Can you work these out from the model? Positions are in its coordinate system, mm. A direction names the side the tool comes from. Give positions to 0.01 mm unless a question says otherwise; leave off trailing zeros. Loops run counter-clockwise (first coordinate to the right, second up) from the corner with the lowest first, then second, coordinate; pieces in that order, holes last. Notation, with made-up numbers: (48.25, 86.25) -> (91.25, 86.25) arc R20 cw to (91.25, 118.25) -> close; hole circle Ø9 at (30.25, 83.25). An arc over 180 degrees is marked (long way). One line per question, with ' | ' between items.
from build123d import *

# Parameters (mm, degrees)
SKETCH1_W                                 = 95
SKETCH1_H                                 = 134
BOSS_EXTRUDE1_DEPTH                       = 2
CSK_FOR_4_FLAT_HEAD_MACHINE_SCREW_2_COUNT = 2
CSK_FOR_4_FLAT_HEAD_MACHINE_SCREW_2_PITCH = 46.7
CSK_FOR_4_FLAT_HEAD_MACHINE_SCREW_3_COUNT = 2
CSK_FOR_4_FLAT_HEAD_MACHINE_SCREW_3_PITCH = 55.505765466
CSK_FOR_4_FLAT_HEAD_MACHINE_SCREW_4_COUNT = 2
CSK_FOR_4_FLAT_HEAD_MACHINE_SCREW_4_PITCH = 30
CSK_FOR_4_FLAT_HEAD_MACHINE_SCREW_5_COUNT = 2
CSK_FOR_4_FLAT_HEAD_MACHINE_SCREW_5_PITCH = 116.985137945
CSK_FOR_4_FLAT_HEAD_MACHINE_SCREW_6_COUNT = 2
CSK_FOR_4_FLAT_HEAD_MACHINE_SCREW_6_PITCH = 131.458824352
SKETCH13_R                                = 24.6
CUT_EXTRUDE2_DEPTH                        = 165.271117364
SKETCH14_R                                = 3
BOSS_EXTRUDE4_DEPTH                       = 19.3
SKETCH15_R                                = 1.15
CUT_EXTRUDE3_DEPTH                        = 15
SKETCH16_W                                = 4
SKETCH16_H                                = 14
CUT_EXTRUDE4_DEPTH                        = 166.388905311


with BuildPart() as part:
    # Sketch1 → Boss-Extrude1 (new body)
    with BuildSketch(Plane.XY):
        with Locations((47.5, 67)):
            Rectangle(SKETCH1_W, SKETCH1_H)
    extrude(amount=BOSS_EXTRUDE1_DEPTH)

    # Sketch8 → CSK for #4 Flat Head Machine Screw (100)2 (revolve, cut)
    with BuildSketch(Plane(origin=(70.85, 130, 0), x_dir=(0, 1, 0), z_dir=(1, 0, 0))):
        Polygon((0, 0), (0, 2), (1.63195, 2), (1.63195, 1.028358553), (2.8575, 0), align=None)
    csk_for_4_flat_head_machine_screw_100 = revolve(axis=Axis((70.85, 130, -6.35), (0, 0, 1)), mode=Mode.SUBTRACT)

    # CSK for _4 Flat Head Machine Screw _ 2: CSK for #4 Flat Head Machine Screw (100)2 ×2
    with Locations(*[(-i * CSK_FOR_4_FLAT_HEAD_MACHINE_SCREW_2_PITCH, 0, 0) for i in range(1, CSK_FOR_4_FLAT_HEAD_MACHINE_SCREW_2_COUNT)]):
        add(csk_for_4_flat_head_machine_screw_100, mode=Mode.SUBTRACT)

    # CSK for _4 Flat Head Machine Screw _ 3: CSK for #4 Flat Head Machine Screw (100)2 ×2
    with Locations(*[Vector(-0.8413540396691381, -0.540484393791738, 0) * (i * CSK_FOR_4_FLAT_HEAD_MACHINE_SCREW_3_PITCH) for i in range(1, CSK_FOR_4_FLAT_HEAD_MACHINE_SCREW_3_COUNT)]):
        add(csk_for_4_flat_head_machine_screw_100, mode=Mode.SUBTRACT)

    # CSK for _4 Flat Head Machine Screw _ 4: CSK for #4 Flat Head Machine Screw (100)2 ×2
    with Locations(*[(0, -i * CSK_FOR_4_FLAT_HEAD_MACHINE_SCREW_4_PITCH, 0) for i in range(1, CSK_FOR_4_FLAT_HEAD_MACHINE_SCREW_4_COUNT)]):
        add(csk_for_4_flat_head_machine_screw_100, mode=Mode.SUBTRACT)

    # CSK for _4 Flat Head Machine Screw _ 5: CSK for #4 Flat Head Machine Screw (100)2 ×2
    with Locations(*[Vector(0.12950362982970207, -0.991578947870986, 0) * (i * CSK_FOR_4_FLAT_HEAD_MACHINE_SCREW_5_PITCH) for i in range(1, CSK_FOR_4_FLAT_HEAD_MACHINE_SCREW_5_COUNT)]):
        add(csk_for_4_flat_head_machine_screw_100, mode=Mode.SUBTRACT)

    # CSK for _4 Flat Head Machine Screw _ 6: CSK for #4 Flat Head Machine Screw (100)2 ×2
    with Locations(*[Vector(-0.47048952632046626, -0.8824055788710445, 0) * (i * CSK_FOR_4_FLAT_HEAD_MACHINE_SCREW_6_PITCH) for i in range(1, CSK_FOR_4_FLAT_HEAD_MACHINE_SCREW_6_COUNT)]):
        add(csk_for_4_flat_head_machine_screw_100, mode=Mode.SUBTRACT)

    # Sketch13 → Cut-Extrude2 (cut, through all)
    with BuildSketch(Plane(origin=(0, 0, 0), x_dir=(-1, 0, 0), z_dir=(0, 0, -1))):
        with Locations((-47.5, 45.5)):
            Circle(SKETCH13_R)
    extrude(amount=-CUT_EXTRUDE2_DEPTH, mode=Mode.SUBTRACT)

    # Sketch14 → Boss-Extrude4 (add)
    with BuildSketch(Plane(origin=(0, 0, 0), x_dir=(-1, 0, 0), z_dir=(0, 0, -1))):
        with Locations((-72, 70.1)):
            Circle(SKETCH14_R)
        with Locations((-23, 70.1)):
            Circle(SKETCH14_R)
        with Locations((-72, 20.9)):
            Circle(SKETCH14_R)
        with Locations((-23, 20.9)):
            Circle(SKETCH14_R)
    extrude(amount=BOSS_EXTRUDE4_DEPTH)

    # Sketch15 → Cut-Extrude3 (cut)
    with BuildSketch(Plane(origin=(0, 0, -19.3), x_dir=(-1, 0, 0), z_dir=(0, 0, -1))):
        with Locations((-72, 70.1)):
            Circle(SKETCH15_R)
        with Locations((-23, 70.1)):
            Circle(SKETCH15_R)
        with Locations((-23, 20.9)):
            Circle(SKETCH15_R)
        with Locations((-72, 20.9)):
            Circle(SKETCH15_R)
    extrude(amount=-CUT_EXTRUDE3_DEPTH, mode=Mode.SUBTRACT)

    # Sketch16 → Cut-Extrude4 (cut, through all)
    with BuildSketch(Plane(origin=(0, 0, 0), x_dir=(-1, 0, 0), z_dir=(0, 0, -1))):
        with Locations((-19, 7)):
            Rectangle(SKETCH16_W, SKETCH16_H)
    extrude(amount=-CUT_EXTRUDE4_DEPTH, mode=Mode.SUBTRACT)


solid = part.part
Q1. If we section it at D-D (y = 65.5): Write out the boundary of the cut face in (x, z), plus the area to 3 significant figures.
Entries:
outline: (0, 0) -> (33.18, 0) -> (33.18, 2) -> (0, 2) -> close; (61.82, 0) -> (95, 0) -> (95, 2) -> (61.82, 2) -> close | area: 133 mm²
Q2. For pin 1 Ø2 at (x, y) = (11, 85.5) entering from -Z; pin 2 Ø5 at (y, z) = (70, -9.5) entering from -X; pin 3 Ø1.8 at (x, y) = (23, 21) entering from -Z; pin 4 Ø2 at (x, y) = (9, 14) entering from +Z, each with a flat end and sliding along its axis, tell me the tip position at first contact or that it passes through.
Entries:
pin 1: z = 0 | pin 2: x = 20 | pin 3: z = -4.3 | pin 4: through
Q3. If we section it at B-B (x = 9): Write out the boundary of the cut face in (y, z), plus the area to 3 significant figures.
Entries:
outline: (0, 0) -> (11.14, 0) -> (12.37, 1.03) -> (12.37, 2) -> (0, 2) -> close; (15.63, 1.03) -> (16.86, 0) -> (134, 0) -> (134, 2) -> (15.63, 2) -> close | area: 260 mm²
Q4. If I drill on probe 1 along X at (y, z) = (130, 1.35); probe 2 along Y at (x, z) = (23, -8.5); probe 3 along Z at (x, y) = (14, 41.5), over which ranges is the centre line in solid material (lowest first)? Write a range as from..to.
Entries:
probe 1: 0..22.52, 25.78..69.22, 72.48..95 | probe 2: 17.9..19.75, 22.05..23.9, 67.1..68.95, 71.25..73.1 | probe 3: 0..2
Q5. On a 3-axis mill with a long thin cutter (end or side, diameter ignored), from which of +Z, -Z, +X, -X, +Y, -Y can I reach the whole of each face in a straight line? I mean faces 1 (the face through (84.897, 12.797, 1.507)), 2 (the face through (23.391, 73.074, -9.515)). Say none if no direction works.
Entries:
face 1: +Z, -Z | face 2: -Z
Q6. If we mould it in two halves opening along Y, with no side actions, what happens to faces 3 (the face through (71, 20, -19.3)), 4 (the face through (69.747, 98.797, 1.507))? For each: pulls with the +Y half, pulls with the -Y half, needs draft (parallel to the pull), parting line crosses it, or undercut.
Entries:
face 3: needs draft | face 4: undercut
Q7. If we section it at C-C (y = 100): Write out the boundary of the cut face in (x, z), plus the area to 3 significant figures.
Entries:
outline: (0, 0) -> (21.29, 0) -> (22.52, 1.03) -> (22.52, 2) -> (0, 2) -> close; (25.78, 1.03) -> (27.01, 0) -> (67.99, 0) -> (69.22, 1.03) -> (69.22, 2) -> (25.78, 2) -> close; (72.48, 1.03) -> (73.71, 0) -> (95, 0) -> (95, 2) -> (72.48, 2) -> close | area: 174 mm²
Q8. If we section it at A-A (z = -10.75): Write out the boundary of the cut face in (x, y), plus the area to 3 significant figures.
Entries:
outline: circle Ø6 at (23, 20.9); circle Ø6 at (23, 70.1); circle Ø6 at (72, 20.9); circle Ø6 at (72, 70.1); hole circle Ø2.3 at (23, 20.9); hole circle Ø2.3 at (23, 70.1); hole circle Ø2.3 at (72, 20.9); hole circle Ø2.3 at (72, 70.1) | area: 96.5 mm²
